```python
from build123d import *

# Parameters (mm, degrees)
SKETCH1_W            = 22
SKETCH1_H            = 58
BOSS_EXTRUDE1_DEPTH  = 2.54
EXTRUDE_THIN2_DEPTH  = 22
SKETCH7_R            = 7.9375
SKETCH7_R_2          = 5.3975
BOSS_EXTRUDE2_DEPTH  = 10.16
SKETCH8_R            = 5.3975
CUT_EXTRUDE1_DEPTH   = 34.515518794
M4_CLEARANCE_HOLE1_D = 4.5


with BuildPart() as part:
    # Sketch1 → Boss-Extrude1 (new body)
    with BuildSketch(Plane.XY):
        Rectangle(SKETCH1_W, SKETCH1_H)
    extrude(amount=BOSS_EXTRUDE1_DEPTH)

    # Sketch6 → Extrude-Thin2 (add)
    with BuildSketch(Plane.ZY.offset(11)):
        Polygon((0, 21.25), (-10.16, 21.25), (-10.16, -21.25), (0, -21.25), (0, -18.71), (-7.62, -18.71), (-7.62, 18.71), (0, 18.71), align=None)
    extrude(amount=-EXTRUDE_THIN2_DEPTH)

    # Sketch7 → Boss-Extrude2 (add)
    with BuildSketch(Plane(origin=(0, 0, -10.16), x_dir=(-1, 0, 0), z_dir=(0, 0, -1))):
        with Locations(Location((0, 9.4592, 0), (0, 0, 90))):
            Circle(SKETCH7_R)
        with Locations(Location((0, 9.4592, 0), (0, 0, 90))):
            Circle(SKETCH7_R_2, mode=Mode.SUBTRACT)
    extrude(amount=-BOSS_EXTRUDE2_DEPTH)

    # Sketch8 → Cut-Extrude1 (cut, through all)
    with BuildSketch(Plane(origin=(0, 0, -10.16), x_dir=(-1, 0, 0), z_dir=(0, 0, -1))):
        with Locations(Location((0, 9.4592, 0), (0, 0, 90))):
            Circle(SKETCH8_R)
    extrude(amount=-CUT_EXTRUDE1_DEPTH, mode=Mode.SUBTRACT)

    # M4 Clearance Hole1 (through all)
    with Locations(Plane(origin=(0, 0, 0), x_dir=(-1, 0, 0), z_dir=(0, 0, -1))):
        with Locations((-5, 24.75), (5, 24.75), (-5, -24.75), (5, -24.75)):
            Hole(M4_CLEARANCE_HOLE1_D / 2)


solid = part.part
```
Work out the finished part from the listing and answer in its coordinate system (mm). A direction names the side the tool comes from. Give positions to 0.01 mm unless a question says otherwise; leave off trailing zeros. Loops run counter-clockwise (first coordinate to the right, second up) from the corner with the lowest first, then second, coordinate; pieces in that order, holes last. Notation, with made-up numbers: (72.5, 48.5) - (107.5, 48.5) arc R22 ccw to (107.5, 65.5) - close; hole circle Ø10 at (-11.75, 68.5). An arc over 180 degrees is marked (long way). One line per question, with ' | ' between items.
(1) The part is cut by section D-D (x = -4.5). Write down the section's boundary in (y, z).
Recorded:
outline: (-29, 0) - (-26.94, 0) - (-26.94, 2.54) - (-29, 2.54) - close; (-22.56, 0) - (-21.25, 0) - (-21.25, -10.16) - (6.48, -10.16) - (6.48, 2.54) - (-22.56, 2.54) - close; (12.44, -10.16) - (21.25, -10.16) - (21.25, 0) - (22.56, 0) - (22.56, 2.54) - (12.44, 2.54) - close; (26.94, 0) - (29, 0) - (29, 2.54) - (26.94, 2.54) - close; hole (-18.71, -7.62) - (2.92, -7.62) - (2.92, 0) - (-18.71, 0) - close; hole (16, -7.62) - (18.71, -7.62) - (18.71, 0) - (16, 0) - close
(2) The part is cut by section C-C (y = 24.75). Write down the section's boundary in (x, z), then the cut area to 3 significant figures.
Recorded:
outline: (-11, 0) - (-7.25, 0) - (-7.25, 2.54) - (-11, 2.54) - close; (-2.75, 0) - (2.75, 0) - (2.75, 2.54) - (-2.75, 2.54) - close; (7.25, 0) - (11, 0) - (11, 2.54) - (7.25, 2.54) - close | area: 33.0 mm²
(3) Each of these flat-tipped pins is pushed along its axis until it touches: pin 1 Ø6 at (x, y) = (5, 24.75) entering from -Z; pin 2 Ø6 at (x, z) = (-0.5, -5.5) entering from +Y; pin 3 Ø2 at (x, z) = (-5.5, -7) entering from -Y. Where does it stop, or does it pass through?
Recorded:
pin 1: stops at z = 0 | pin 2: stops at y = 21.25 | pin 3: stops at y = -21.25
(4) The part is cut by section A-A (x = 0). Write down the section's boundary in (y, z), then the cut area to 3 significant figures.
Recorded:
outline: (-29, 0) - (-21.25, 0) - (-21.25, -10.16) - (4.06, -10.16) - (4.06, 2.54) - (-29, 2.54) - close; (14.86, -10.16) - (21.25, -10.16) - (21.25, 0) - (29, 0) - (29, 2.54) - (14.86, 2.54) - close; hole (-18.71, -7.62) - (1.52, -7.62) - (1.52, 0) - (-18.71, 0) - close; hole (17.4, -7.62) - (18.71, -7.62) - (18.71, 0) - (17.4, 0) - close | area: 278 mm²
(5) The mould has two halves that part along X. Classify faces 4 (the face through (-3.04, 16.79, -3.86)), 5 (the face through (5, -27, 1)), 6 (the face through (0, 18.71, -4)): +X half, -X half, draft (parallel to the pull), parting line (faces both ways), or undercut.
Recorded:
face 4: parting line | face 5: undercut | face 6: draft
(6) The part is cut by section B-B (z = -4.25). Count the separate pieces of the cut face and the enclosed holes in it, then the cut area to 3 significant figures.
Recorded:
separate pieces: 3 | enclosed holes: 1 | area: 218 mm²
(7) Straight lines are drawn through the part: probe 1 along Z at (x, y) = (-9.75, 3); probe 2 along Y at (x, z) = (-8.25, -3.75); probe 3 along Y at (x, z) = (5, 1.15). For each, find the intervals that lie inside material, in ascending order.
Recorded:
probe 1: z = -10.16 to -7.62, 0 to 2.54 | probe 2: y = -21.25 to -18.71, 18.71 to 21.25 | probe 3: y = -29 to -27, -22.5 to 7.43, 11.49 to 22.5, 27 to 29
(8) A tool of negligible diameter and unlimited length cuts with its end or side. For faces 1 (the face through (0, 21.25, -5)), 2 (the face through (0, -18.71, -4)), 3 (the face through (0, -21.25, -5)), from which of +Z, -Z, +X, -X, +Y, -Y can it reach the whole face along a straight path? Write none if from no direction.
Recorded:
face 1: -Z, +X, -X, +Y | face 2: +X, -X | face 3: -Z, +X, -X, -Y
